from build123d import *

# Parameters (mm, degrees)
PAD010_DEPTH     = 18
SKETCH020_W      = 17.45
SKETCH020_H      = 2.4
POCKET011_DEPTH  = 6.75
SKETCH021_W      = 6
SKETCH021_H      = 6
PAD011_DEPTH     = 0.75
SKETCH022_W      = 4
SKETCH022_H      = 9.5
POCKET012_DEPTH  = 1
CHAMFER_SIZE     = 1
CHAMFER_FACE23_W = 6
CHAMFER_FACE23_H = 0.75
PAD012_DEPTH     = 12
PAD013_DEPTH     = 0.75
PAD014_DEPTH     = 0.5


with BuildPart() as part:
    # Sketch019 → Pad010 (new body)
    with BuildSketch(Plane.XZ):
        Polygon((21.151384, 8.480667), (15.151384, 9.360667), (15.151384, 8.760667), (6.701384, 10), (6.701384, 5.25), (5.201384, 5.25), (5.201384, 4.25), (22.651384, 4.25), (22.651384, 5.25), (21.151384, 5.25), align=None)
    extrude(amount=PAD010_DEPTH)

    # Sketch020 → Pocket011 (cut)
    with BuildSketch(Plane.XY.offset(12)):
        with Locations((13.926384, -9)):
            Rectangle(SKETCH020_W, SKETCH020_H)
    extrude(amount=-POCKET011_DEPTH, mode=Mode.SUBTRACT)

    # Sketch021 (on Face11 of Pocket011) → Pad011 (join)
    with BuildSketch(Plane(origin=(0, 0, 4.25), x_dir=(1, 0, 0), z_dir=(0, 0, -1))):
        with Locations((8.201384, 3)):
            Rectangle(SKETCH021_W, SKETCH021_H)
    extrude(amount=PAD011_DEPTH)

    # Sketch022 (on Face13 of Pad011) → Pocket012 (cut)
    with BuildSketch(Plane(origin=(0, 0, 4.25), x_dir=(1, 0, 0), z_dir=(0, 0, -1))):
        with Locations((20.651384, 9)):
            Rectangle(SKETCH022_W, SKETCH022_H)
    extrude(amount=-POCKET012_DEPTH, mode=Mode.SUBTRACT)

    # Chamfer
    chamfer_edges = [part.edges().sort_by_distance(p)[0] for p in [
        (18.651384, -4.25, 4.75),
        (18.651384, -13.75, 4.75),
        (22.651384, -4.25, 4.75),
        (22.651384, -13.75, 4.75),
    ]]
    chamfer(chamfer_edges, length=CHAMFER_SIZE)

    # Chamfer Face23 → Pad012 (add)
    with BuildSketch(Plane(origin=(8.201384, -6, 3.875), x_dir=(-1, 0, 0), z_dir=(0, -1, 0))):
        Rectangle(CHAMFER_FACE23_W, CHAMFER_FACE23_H)
    extrude(amount=PAD012_DEPTH)

    # Pad012 Face7 → Pad013 (add)
    with BuildSketch(Plane(origin=(16.064496, -9, 4.25), x_dir=(0, -1, 0), z_dir=(0, 0, -1))):
        Polygon((-5.75, -6.586888), (-4.75, -5.586888), (-4.75, -3.586888), (-3.75, -2.586888), (3.75, -2.586888), (4.75, -3.586888), (4.75, -5.586888), (5.75, -6.586888), (9, -6.586888), (9, 4.863112), (-9, 4.863112), (-9, -6.586888), align=None)
    extrude(amount=PAD013_DEPTH)

    # Pad013 Face25 → Pad014 (add)
    with BuildSketch(Plane(origin=(12.988741, -9, 3.5), x_dir=(0, -1, 0), z_dir=(0, 0, -1))):
        Polygon((-5.75, -9.662643), (-4.75, -8.662643), (-4.75, -6.662643), (-3.75, -5.662643), (3.75, -5.662643), (4.75, -6.662643), (4.75, -8.662643), (5.75, -9.662643), (9, -9.662643), (9, 7.787357), (-9, 7.787357), (-9, -9.662643), align=None)
    extrude(amount=PAD014_DEPTH)


with BuildPart() as part_1:
    # Body004 placement: moved
    add(part.part.moved(Location((0, -37.5, 0))))


solid = part_1.part
Check sheet for the modelled part. Datum: model origin and axes. Units: mm. A direction names the side the tool comes from. Give positions to 0.01 mm unless a question says otherwise; leave off trailing zeros. Write each loop counter-clockwise with the first axis right and the second up, starting at its lowest first coordinate (ties: lowest second). Pieces come first, ordered by that corner, then holes. Notation, with made-up numbers: (36, 54.25) -> (70, 54.25) arc R10 cw to (70, 63.25) -> close; hole circle Ø10 at (23.5, 31). An arc over 180 degrees is marked (long way). One line per item, written item: value. Start each with the question number.
Item 1: Tool access check on faces 4 (the flat face through (22.1, -51.7, 4.1)), 5 (the flat face through (22, -53, 5.25)), 6 (the flat face through (19.1, -50.7, 4.1)), 7 (the flat face through (6.701, -41, 8)). Record the directions out of +Z, -Z, +X, -X, +Y, -Y that give a thin tool (end or side, any length) a straight path to the whole face; none if there is none.
Item 2: Material ranges on probe 1 along Y at (x, z) = (11.75, 9); probe 2 along X at (y, z) = (-48.25, 3.5); probe 3 along X at (y, z) = (-49.5, 7.25), recorded low to high. Write a range as from..to.
Item 3: Section check B-B on y = -44. Record the cut outline in (x, z).
Item 4: Section check C-C on x = 9. Record the cut outline in (y, z), then the cut area to 3 significant figures.
Item 5: Gauge pin test, flat ends, axial feed: pin 1 (1.5 mm diameter, centred on y = -51.5, z = 9, fed in from +X); pin 2 (1.2 mm diameter, centred on x = 22.5, y = -39.5, fed in from +Z); pin 3 (2 mm diameter, centred on x = 10, y = -40, fed in from +Z). Record the tip position at first contact, or that the pin passes through.
Item 6: Section check D-D on z = 5. Record the cut outline in (x, y).
Item 7: Draft check along Y on faces 1 (the flat face through (14, -45.3, 7)), 2 (the flat face through (14, -37.5, 6)), 3 (the flat face through (5.201, -47, 4)). Enter one of: +Y half, -Y half, draft (parallel to the pull), parting line (faces both ways), or undercut.
Item 8: Section check A-A on z = 8. Record the cut outline in (x, y).
Results list:
1. face 4: +Z, -Z, +X
1. face 5: +Z, +X, +Y, -Y
1. face 6: -Z, +X
1. face 7: +Z, -X, +Y, -Y
2. probe 1: -55.5..-47.7, -45.3..-37.5
2. probe 2: 5.2..18.65
2. probe 3: 6.7..21.15
3. outline: (5.2, 3) -> (18.65, 3) -> (18.65, 5.25) -> (21.15, 5.25) -> (21.15, 8.48) -> (15.15, 9.36) -> (15.15, 8.76) -> (6.7, 10) -> (6.7, 5.25) -> (5.2, 5.25) -> close
4. outline: (-55.5, 3) -> (-37.5, 3) -> (-37.5, 9.66) -> (-45.3, 9.66) -> (-45.3, 5.25) -> (-47.7, 5.25) -> (-47.7, 9.66) -> (-55.5, 9.66) -> close
4. area: 109 mm²
5. pin 1: x = 21.15
5. pin 2: z = 5.25
5. pin 3: z = 9.66
6. outline: (5.2, -55.5) -> (22.65, -55.5) -> (22.65, -52.25) -> (21.65, -51.25) -> (19.65, -51.25) -> (18.65, -50.25) -> (18.65, -42.75) -> (19.65, -41.75) -> (21.65, -41.75) -> (22.65, -40.75) -> (22.65, -37.5) -> (5.2, -37.5) -> close
7. face 1: undercut
7. face 2: +Y half
7. face 3: draft
8. outline: (6.7, -55.5) -> (21.15, -55.5) -> (21.15, -47.7) -> (6.7, -47.7) -> close; (6.7, -45.3) -> (21.15, -45.3) -> (21.15, -37.5) -> (6.7, -37.5) -> close
